Geometry: final body of the model. Coordinates: model frame, mm. Face numbers are marked on the shaded views. Round coordinates to 2 decimals unless told otherwise and drop trailing zeros. Loops run counter-clockwise (first coordinate to the right, second up) from the corner with the lowest first, then second, coordinate; pieces in that order, holes last. Notation, with made-up numbers: (-31.75, -23.75) - (-25.75, -23.75) arc R22 cw to (-25.75, -10.75) - close; hole circle Ø2 at (53, 18). An arc over 180 degrees is marked (long way). Return JSON: item names as keys, results as strings. Group by question number.
1. Draft query along Y for the marked faces 1, 2 and 3. Return one class per face: +Y half, -Y half, draft (parallel to the pull), parting line (faces both ways), or undercut.
2. Section A-A on x = 0. Return loops of the section in (y, z).
3. First-contact query: pin 1 Ø6 at (x, y) = (0, 200) entering from +Z; pin 2 Ø3.5 at (x, y) = (0, 7.5) entering from +Z. Flat tips, straight axial feed; report the tip coordinate or a pass-through.
4. Material intervals for probe 1 along X at (y, z) = (200, 0); probe 2 along X at (y, z) = (101.5, -0.25), sorted ascending.
5. Section B-B on y = 7.5. Return loops of the section in (x, z).
6. Section C-C on z = 4. Return loops of the section in (x, y), and give its area (3 significant figures).
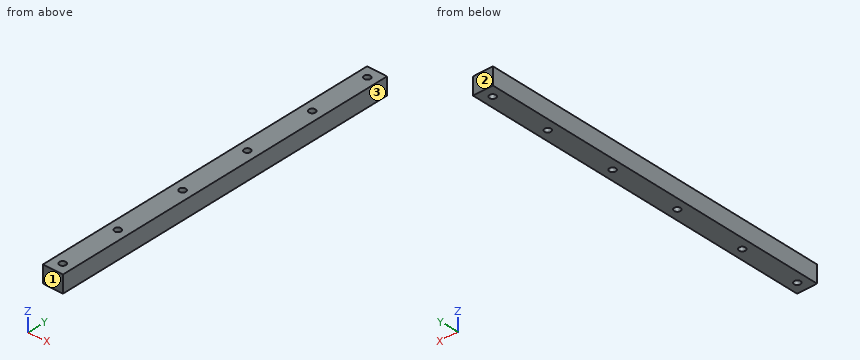
from build123d import *

# Parameters (mm, degrees)
SKETCH1_W           = 14
SKETCH1_H           = 12
BOSS_EXTRUDE1_DEPTH = 250
SKETCH2_R           = 2.25
CUT_EXTRUDE1_DEPTH  = 6
CUT_EXTRUDE2_REACH  = 252.386
SKETCH3_R           = 2.25


with BuildPart() as part:
    # Sketch1 → Boss-Extrude1 (new body)
    with BuildSketch(Plane(origin=(0, 0, 0), x_dir=(1, 0, 0), z_dir=(0, 1, 0))):
        Rectangle(SKETCH1_W, SKETCH1_H)
    extrude(amount=BOSS_EXTRUDE1_DEPTH)

    # Sketch2 → Cut-Extrude1 (cut, symmetric)
    with BuildSketch(Plane.XY):
        with Locations((0, 7.5)):
            Circle(SKETCH2_R)
        with Locations((0, 242.5)):
            Circle(SKETCH2_R)
    extrude(amount=CUT_EXTRUDE1_DEPTH, both=True, mode=Mode.SUBTRACT)

    # Sketch3 → Cut-Extrude2 (cut, up to next)
    with BuildSketch(Plane(origin=(0, 0, -6), x_dir=(-1, 0, 0), z_dir=(0, 0, -1)), mode=Mode.PRIVATE) as cut_extrude2_sk1:
        with Locations((0, 200)):
            Circle(SKETCH3_R)
    cut_extrude2_tool1 = extrude(cut_extrude2_sk1.sketch, amount=-CUT_EXTRUDE2_REACH, mode=Mode.PRIVATE) & part.part
    # Sketch3 → Cut-Extrude2 (cut, up to next)
    with BuildSketch(Plane(origin=(0, 0, -6), x_dir=(-1, 0, 0), z_dir=(0, 0, -1)), mode=Mode.PRIVATE) as cut_extrude2_sk2:
        with Locations((0, 150)):
            Circle(SKETCH3_R)
    cut_extrude2_tool2 = extrude(cut_extrude2_sk2.sketch, amount=-CUT_EXTRUDE2_REACH, mode=Mode.PRIVATE) & part.part
    # Sketch3 → Cut-Extrude2 (cut, up to next)
    with BuildSketch(Plane(origin=(0, 0, -6), x_dir=(-1, 0, 0), z_dir=(0, 0, -1)), mode=Mode.PRIVATE) as cut_extrude2_sk3:
        with Locations((0, 100)):
            Circle(SKETCH3_R)
    cut_extrude2_tool3 = extrude(cut_extrude2_sk3.sketch, amount=-CUT_EXTRUDE2_REACH, mode=Mode.PRIVATE) & part.part
    # Sketch3 → Cut-Extrude2 (cut, up to next)
    with BuildSketch(Plane(origin=(0, 0, -6), x_dir=(-1, 0, 0), z_dir=(0, 0, -1)), mode=Mode.PRIVATE) as cut_extrude2_sk4:
        with Locations((0, 50)):
            Circle(SKETCH3_R)
    cut_extrude2_tool4 = extrude(cut_extrude2_sk4.sketch, amount=-CUT_EXTRUDE2_REACH, mode=Mode.PRIVATE) & part.part
    add(cut_extrude2_tool1.solids().sort_by_distance((0, 200, -6))[0], mode=Mode.SUBTRACT)
    add(cut_extrude2_tool2.solids().sort_by_distance((0, 150, -6))[0], mode=Mode.SUBTRACT)
    add(cut_extrude2_tool3.solids().sort_by_distance((0, 100, -6))[0], mode=Mode.SUBTRACT)
    add(cut_extrude2_tool4.solids().sort_by_distance((0, 50, -6))[0], mode=Mode.SUBTRACT)


solid = part.part
Taken from the geometry:
{
 "1": {"face 1": "-Y half", "face 2": "+Y half", "face 3": "draft"},
 "2": {"outline": "(0, -6) - (5.25, -6) - (5.25, 6) - (0, 6) - close; (9.75, -6) - (47.75, -6) - (47.75, 6) - (9.75, 6) - close; (52.25, -6) - (97.75, -6) - (97.75, 6) - (52.25, 6) - close; (102.25, -6) - (147.75, -6) - (147.75, 6) - (102.25, 6) - close; (152.25, -6) - (197.75, -6) - (197.75, 6) - (152.25, 6) - close; (202.25, -6) - (240.25, -6) - (240.25, 6) - (202.25, 6) - close; (244.75, -6) - (250, -6) - (250, 6) - (244.75, 6) - close"},
 "3": {"pin 1": "z = 6", "pin 2": "through"},
 "4": {"probe 1": "-7 to -2.25, 2.25 to 7", "probe 2": "-7 to -1.68, 1.68 to 7"},
 "5": {"outline": "(-7, -6) - (-2.25, -6) - (-2.25, 6) - (-7, 6) - close; (2.25, -6) - (7, -6) - (7, 6) - (2.25, 6) - close"},
 "6": {"outline": "(-7, 0) - (7, 0) - (7, 250) - (-7, 250) - close; hole circle Ø4.5 at (0, 7.5); hole circle Ø4.5 at (0, 50); hole circle Ø4.5 at (0, 100); hole circle Ø4.5 at (0, 150); hole circle Ø4.5 at (0, 200); hole circle Ø4.5 at (0, 242.5)", "area": "3,400 mm2"}
}
